```python
from build123d import *

# Parameters (mm, degrees)
ESQUISSE2_W             = 260
ESQUISSE2_H             = 130
BOSS_EXTRU_2_DEPTH      = 70
ESQUISSE3_R             = 45
ENL_V_MAT_EXTRU_1_DEPTH = 12
CONG_1_R                = 2
ESQUISSE4_R             = 12.5
ENL_V_MAT_EXTRU_2_DEPTH = 38
CONG_2_R                = 2
CONG_3_R                = 2
CONG_4_R                = 10
CONG_5_R                = 10
CONG_6_R                = 10
CONG_7_R                = 10
ESQUISSE6_R             = 10
ENL_V_MAT_EXTRU_3_DEPTH = 71


with BuildPart() as part:
    # Esquisse2 → Boss.-Extru.2 (new body)
    with BuildSketch(Plane(origin=(0, 0, 0), x_dir=(1, 0, 0), z_dir=(0, 1, 0))):
        Rectangle(ESQUISSE2_W, ESQUISSE2_H)
    extrude(amount=BOSS_EXTRU_2_DEPTH)

    # Esquisse3 → Enlèv. mat.-Extru.1 (cut)
    with BuildSketch(Plane(origin=(0, 70, 0), x_dir=(1, 0, 0), z_dir=(0, 1, 0))):
        with Locations((-65, 0)):
            Circle(ESQUISSE3_R)
    extrude(amount=-ENL_V_MAT_EXTRU_1_DEPTH, mode=Mode.SUBTRACT)

    # Congé1
    cong_1_edges = [part.edges().sort_by_distance(p)[0] for p in [
        (-110, 58, 0),
    ]]
    fillet(cong_1_edges, radius=CONG_1_R)

    # Esquisse4 → Enlèv. mat.-Extru.2 (cut)
    with BuildSketch(Plane(origin=(0, 58, 0), x_dir=(1, 0, 0), z_dir=(0, 1, 0))):
        with Locations((-65, 0)):
            Circle(ESQUISSE4_R)
    extrude(amount=-ENL_V_MAT_EXTRU_2_DEPTH, mode=Mode.SUBTRACT)

    # Congé2
    cong_2_edges = [part.edges().sort_by_distance(p)[0] for p in [
        (-77.5, 58, 0),
    ]]
    fillet(cong_2_edges, radius=CONG_2_R)

    # Congé3
    cong_3_edges = [part.edges().sort_by_distance(p)[0] for p in [
        (-77.5, 20, 0),
    ]]
    fillet(cong_3_edges, radius=CONG_3_R)

    # Congé4
    cong_4_edges = [part.edges().sort_by_distance(p)[0] for p in [
        (-130, 35, -65),
    ]]
    fillet(cong_4_edges, radius=CONG_4_R)

    # Congé5
    cong_5_edges = [part.edges().sort_by_distance(p)[0] for p in [
        (-130, 35, 65),
    ]]
    fillet(cong_5_edges, radius=CONG_5_R)

    # Congé6
    cong_6_edges = [part.edges().sort_by_distance(p)[0] for p in [
        (130, 35, 65),
    ]]
    fillet(cong_6_edges, radius=CONG_6_R)

    # Congé7
    cong_7_edges = [part.edges().sort_by_distance(p)[0] for p in [
        (130, 35, -65),
    ]]
    fillet(cong_7_edges, radius=CONG_7_R)

    # Esquisse6 → Enlèv. mat.-Extru.3 (cut, through all)
    with BuildSketch(Plane(origin=(0, 70, 0), x_dir=(1, 0, 0), z_dir=(0, 1, 0))):
        with Locations((10, 45)):
            Circle(ESQUISSE6_R)
        with Locations((10, -45)):
            Circle(ESQUISSE6_R)
    extrude(amount=-ENL_V_MAT_EXTRU_3_DEPTH, mode=Mode.SUBTRACT)


solid = part.part
```
Input: part model. Units: mm. Frame: model coordinates. A direction names the side the tool comes from. Round coordinates to 2 decimals unless told otherwise and drop trailing zeros. Write each loop counter-clockwise with the first axis right and the second up, starting at its lowest first coordinate (ties: lowest second). Pieces come first, ordered by that corner, then holes. Notation, with made-up numbers: (4.25, 46) -> (44.25, 46) arc R24 ccw to (44.25, 57) -> close; hole circle Ø3 at (-20, 58). An arc over 180 degrees is marked (long way). Answer as CSV lines item,"result".
1. Section C-C (z = 48). Return the cut outline in (x, y).
Geometry says:
outline,"(-130, 0) -> (0.46, 0) -> (0.46, 70) -> (-130, 70) -> close; (19.54, 0) -> (130, 0) -> (130, 70) -> (19.54, 70) -> close"
2. Section A-A (x = 4.5). Return the cut outline in (y, z).
Geometry says:
outline,"(0, -65) -> (70, -65) -> (70, -53.35) -> (0, -53.35) -> close; (0, -36.65) -> (70, -36.65) -> (70, 36.65) -> (0, 36.65) -> close; (0, 53.35) -> (70, 53.35) -> (70, 65) -> (0, 65) -> close"
3. Mould query, pull axis Z, two halves, no side actions, for faces 3 (the cylindrical face through (-77.488, 39.238, -0.55)), 4 (the flat face through (-130, 35, 1)), 5 (the flat face through (-2, 35, 65)). Classes: +Z half, -Z half, draft (parallel to the pull), parting line (faces both ways), or undercut.
Geometry says:
face 3,"undercut"
face 4,"draft"
face 5,"+Z half"
4. Section D-D (z = 0). Return the cut outline in (x, y).
Geometry says:
outline,"(-130, 0) -> (130, 0) -> (130, 70) -> (-20, 70) -> (-20, 60) arc R2 cw to (-22, 58) -> (-50.5, 58) arc R2 ccw to (-52.5, 56) -> (-52.5, 22) arc R2 cw to (-54.5, 20) -> (-75.5, 20) arc R2 cw to (-77.5, 22) -> (-77.5, 56) arc R2 ccw to (-79.5, 58) -> (-108, 58) arc R2 cw to (-110, 60) -> (-110, 70) -> (-130, 70) -> close"
5. Section B-B (y = 37). Return the cut outline in (x, z).
Geometry says:
outline,"(-130, -55) arc R10 ccw to (-120, -65) -> (120, -65) arc R10 ccw to (130, -55) -> (130, 55) arc R10 ccw to (120, 65) -> (-120, 65) arc R10 ccw to (-130, 55) -> close; hole circle Ø25 at (-65, 0); hole circle Ø20 at (10, -45); hole circle Ø20 at (10, 45)"
6. Contact query for flat-ended pins moving along their axis: P1, Ø17, axis at x = -62, z = 4, coming from the +Y side; P2, Ø10, axis at x = -95.5, z = -11.5, coming from the +Y side. Output: stop coordinate, or through.
Geometry says:
P1,"stops at y = 57.73"
P2,"stops at y = 58"
7. Reachability of faces 1 (the flat face through (-65, 20, 0)), 2 (the cylindrical face through (-127.15, 35.49, 61.99)) from +Z, -Z, +X, -X, +Y, -Y: full face, straight path, thin tool, end or side. Return the list, or none.
Geometry says:
face 1,"+Y"
face 2,"+Z, -X, +Y, -Y"
8. Ray query, L1, parallel to Z at x = 10, y = 17.5; L2, parallel to Z at x = -65, y = 35; L3, parallel to X at y = 66.75, z = 0. Return the intervals inside material, ascending. Write a range as [from, to].
Geometry says:
L1,"z = [-65, -55], [-35, 35], [55, 65]"
L2,"z = [-65, -12.5], [12.5, 65]"
L3,"x = [-130, -110], [-20, 130]"
